Can you work these out from the model? Positions are in its coordinate system, mm. Face numbers are marked on the shaded views. A direction names the side the tool comes from. Round coordinates to 2 decimals unless told otherwise and drop trailing zeros. Order: outer loops, then holes, each group sorted by start corner. A loop starts at its lowest first (then second) coordinate and runs counter-clockwise, first axis right, second up. Notation, with made-up numbers: (-9, 66.5) - (2, 66.5) arc R28 ccw to (2, 105.5) - close; hole circle Ø10 at (35.5, 53). An arc over 180 degrees is marked (long way). Write item = value, one per line.
Autodesk Inventor part; units mm, degrees
ref_plane "YZ Plane" through (0, 0, 0) normal (1, 0, 0) x (0, 1, 0)
ref_plane "XZ Plane" through (0, 0, 0) normal (0, 1, 0) x (-1, 0, 0)
ref_plane "XY Plane" through (0, 0, 0) normal (0, 0, 1) x (1, 0, 0)
sketch "Sketch1" plane through (0, 0, 0) normal (0, 1, 0) x (-1, 0, 0)
  line L0 (45, 45) -> (-45, 45)
  line L1 (-45, 45) -> (-45, -45)
  line L2 (-45, -45) -> (45, -45)
  line L3 (45, -45) -> (45, 45)
  line L4 (45, 45) -> (-45, -45)
  line L5 (45, -45) -> (-45, 45)
  point P0 (0, 0)
  point P1 (0, 0)
  dimension "d0" = 90
  dimension "d1" = 90
extrude "Extrusion1" add sketch "Sketch1" along normal blind 25
sketch "Sketch5" plane through (0, 25, 0) normal (0, 1, 0) x (1, 0, 0)
  circle A0 centre (0, 0) radius 20.5
  dimension "d27" = 41
extrude "Extrusion3" cut sketch "Sketch5" against normal blind 20
sketch "Sketch6" plane through (0, 5, 0) normal (0, 1, 0) x (1, 0, 0)
  circle A0 centre (0, 0) radius 5
  dimension "d30" = 10
extrude "Extrusion4" cut sketch "Sketch6" against normal blind 20
fillet "Fillet2" radius 5 8 edges at (45, 0, 0) (0, 0, -45) (-45, 0, 0) (0, 0, 45) (45, 25, 0) (0, 25, -45) (-45, 25, 0) (0, 25, 45)
chamfer "Chamfer1" distance 5 angle 45 1 edges at (-20.5, 25, 0)
fillet "Fillet3" radius 5 12 edges at (43.5355, 23.5355, 43.5355) (43.5355, 1.4645, 43.5355) (45, 12.5, 45) (43.5355, 23.5355, -43.5355) (43.5355, 1.4645, -43.5355) (45, 12.5, -45) (-43.5355, 23.5355, 43.5355) (-43.5355, 1.4645, 43.5355) (-45, 12.5, 45) (-45, 12.5, -45) (-43.5355, 1.4645, -43.5355) (-43.5355, 23.5355, -43.5355)
properties part number "supportbalises_3DPrint"
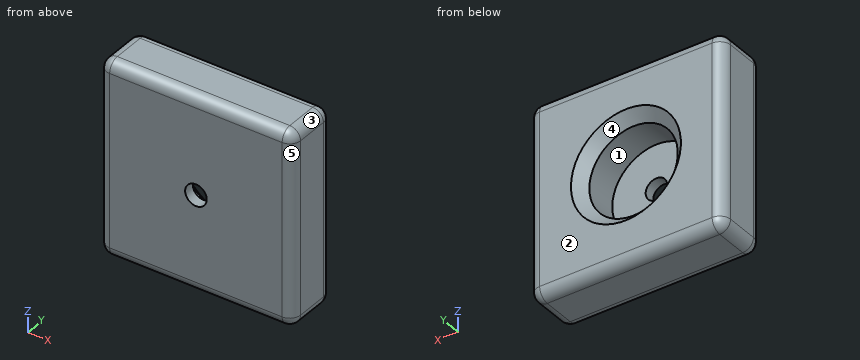
(1) If we section it at A-A (z = 0): Write out the boundary of the cut face in (x, y), plus the area to 3 significant figures.
Computed:
outline = (-45, 5) arc R5 ccw to (-40, 0) - (-5, 0) - (-5, 5) - (-20.5, 5) - (-20.5, 20) - (-25.5, 25) - (-40, 25) arc R5 ccw to (-45, 20) - close; (5, 0) - (40, 0) arc R5 ccw to (45, 5) - (45, 20) arc R5 ccw to (40, 25) - (25.5, 25) - (20.5, 20) - (20.5, 5) - (5, 5) - close
area = 1,330 mm^2
(2) If I drill on line 1 (Z direction, x = -4.5, y = 20.5); line 2 (X direction, y = 11, z = 0); line 3 (Y direction, x = 20.5, z = 40.5), over which ranges is the centre line in solid material (lowest first)? Write a range as from..to.
Computed:
line_1 = -44.97..-20.51, 20.51..44.97
line_2 = -45..-20.5, 20.5..45
line_3 = 0.03..24.97
(3) If we section it at B-B (x = 0): Write out the boundary of the cut face in (y, z), plus the area to 3 significant figures.
Computed:
outline = (0, -40) arc R5 ccw to (5, -45) - (20, -45) arc R5 ccw to (25, -40) - (25, -25.5) - (20, -20.5) - (5, -20.5) - (5, -5) - (0, -5) - close; (0, 5) - (5, 5) - (5, 20.5) - (20, 20.5) - (25, 25.5) - (25, 40) arc R5 ccw to (20, 45) - (5, 45) arc R5 ccw to (0, 40) - close
area = 1,330 mm^2
(4) If we section it at C-C (y = 9.5): Write out the boundary of the cut face in (x, z).
Computed:
outline = (-45, -40) arc R5 ccw to (-40, -45) - (40, -45) arc R5 ccw to (45, -40) - (45, 40) arc R5 ccw to (40, 45) - (-40, 45) arc R5 ccw to (-45, 40) - close; hole circle Ø41 at (0, 0)
(5) On a 3-axis mill with a long thin cutter (end or side, diameter ignored), from which of +Z, -Z, +X, -X, +Y, -Y can I reach the whole of each face in a straight line? I mean the marked faces 1 and 2. Say none if no direction works.
Computed:
face_1 = +Y
face_2 = +Z, -Z, +X, -X, +Y
(6) If we section it at D-D (y = 22.25): Write out the boundary of the cut face in (x, z), plus the area to 3 significant figures.
Computed:
outline = (-44.47, -40) arc R4.47 ccw to (-40, -44.47) - (40, -44.47) arc R4.47 ccw to (44.47, -40) - (44.47, 40) arc R4.47 ccw to (40, 44.47) - (-40, 44.47) arc R4.47 ccw to (-44.47, 40) - close; hole circle Ø45.5 at (0, 0)
area = 6,270 mm^2
(7) Will these pins go through, and if not, where does the flat tip stop? P1, Ø20.5, axis at x = 10, z = 9, coming from the +Y side; P2, Ø6, axis at x = 0, z = 0, coming from the +Y side.
Computed:
P1 = 23.2
P2 = through
(8) Thinking about a two-plate mould opening in Z: for the marked faces 3, 4 and 5, which applies, +Z half, -Z half, draft (parallel to the pull), parting line (faces both ways), or undercut?
Computed:
face_3 = +Z half
face_4 = undercut
face_5 = draft
